from build123d import *

# Parameters (mm, degrees)
SKETCH_1_R      = 1.5
EXTRUDE_1_DEPTH = 1


with BuildPart() as part:
    # 草图1 → 凸台-拉伸1 (new body)
    with BuildSketch(Plane.XY):
        with BuildLine():
            ThreePointArc((9.027564348, -14.530044737), (9.452188044, -14.317284831), (9.814671703, -14.010401047))
            add(Edge.make_bspline(
                [(9.814671703, -14.010401047), (12.18822328, -11.458756692), (15.692863494, -5.893557839), (16.722450019, 0.624994049), (16.609112546, 4.098471157)],
                knots=[0.022064742, 0.022064742, 0.022064742, 0.022064742, 0.499959338, 0.977990906, 0.977990906, 0.977990906, 0.977990906], degree=3))
            ThreePointArc((16.609112546, 4.098471157), (16.53806505, 4.565454975), (16.359479137, 5.002752018))
            add(Edge.make_bspline(
                [(16.359479137, 5.002752018), (14.674806415, 8.042450428), (10.446892996, 13.109630634), (4.583537519, 16.088725104), (1.237093036, 17.061322309)],
                knots=[0.022009094, 0.022009094, 0.022009094, 0.022009094, 0.500040662, 0.977935258, 0.977935258, 0.977935258, 0.977935258], degree=3))
            ThreePointArc((1.237093036, 17.061322309), (0.768508115, 17.138783476), (0.294870912, 17.103571828))
            add(Edge.make_bspline(
                [(0.294870912, 17.103571828), (-3.125200659, 16.434385016), (-9.231172481, 13.992221488), (-13.895447236, 9.324238792), (-15.845236863, 6.448095314)],
                knots=[0.022064742, 0.022064742, 0.022064742, 0.022064742, 0.499960608, 0.977922402, 0.977922402, 0.977922402, 0.977922402], degree=3))
            ThreePointArc((-15.845236863, 6.448095314), (-16.062723303, 6.027327569), (-16.175163145, 5.567215485))
            add(Edge.make_bspline(
                [(-16.175163145, 5.567215485), (-16.595831692, 2.107197873), (-16.160161694, -4.45559692), (-13.161387867, -10.33481003), (-11.028034261, -13.078319909)],
                knots=[0.021996491, 0.021996491, 0.021996491, 0.021996491, 0.499960843, 0.977990945, 0.977990945, 0.977990945, 0.977990945], degree=3))
            ThreePointArc((-11.028034261, -13.078319909), (-10.696067568, -13.414360903), (-10.294548569, -13.663173939))
            add(Edge.make_bspline(
                [(-10.294548569, -13.663173939), (-7.144931204, -15.132114571), (-0.746064836, -16.746443383), (5.74855557, -15.710187793), (9.027564348, -14.530044737)],
                knots=[0.022009307, 0.022009307, 0.022009307, 0.022009307, 0.500040658, 0.977935258, 0.977935258, 0.977935258, 0.977935258], degree=3))
        make_face()
        with Locations((8.264326198, -12.518023506)):
            Circle(SKETCH_1_R, mode=Mode.SUBTRACT)
        with Locations((-9.351530584, -11.728123283)):
            Circle(SKETCH_1_R, mode=Mode.SUBTRACT)
        with Locations((-14.043889946, 5.269644693)):
            Circle(SKETCH_1_R, mode=Mode.SUBTRACT)
        with Locations((0.671929263, 14.984942812)):
            Circle(SKETCH_1_R, mode=Mode.SUBTRACT)
        with Locations((14.459165069, 3.991559284)):
            Circle(SKETCH_1_R, mode=Mode.SUBTRACT)
        with BuildLine():
            ThreePointArc((-12.084118167, 4.284259186), (-11.989009709, 4.498598439), (-11.919642267, 4.722596412))
            add(Edge.make_bspline(
                [(0.333250802, 12.818762133), (-2.935666702, 13.36550918), (-8.291080057, 12.535805727), (-11.122073794, 7.958530689), (-11.919642267, 4.722596412)],
                knots=[0.011876539, 0.011876539, 0.011876539, 0.011876539, 0.500003959, 0.988536873, 0.988536873, 0.988536873, 0.988536873], degree=3))
            ThreePointArc((0.333250802, 12.818762133), (0.573655745, 12.793365714), (0.815368633, 12.797159765))
            add(Edge.make_bspline(
                [(12.293898461, 3.640629682), (11.788818781, 6.932897703), (9.378560044, 11.743845098), (4.119958064, 13.049350775), (0.815368633, 12.797159765)],
                knots=[0.011651073, 0.011651073, 0.011651073, 0.011651073, 0.499978932, 0.988122793, 0.988122793, 0.988122793, 0.988122793], degree=3))
            ThreePointArc((12.293898461, 3.640629682), (12.343962742, 3.407799774), (12.421347321, 3.182571388))
            add(Edge.make_bspline(
                [(7.261467235, -10.567176253), (10.236427241, -9.069498048), (14.068062226, -5.28940284), (13.683697639, 0.116101841), (12.421347321, 3.182571388)],
                knots=[0.011651023, 0.011651023, 0.011651023, 0.011651023, 0.499963297, 0.988308236, 0.988308236, 0.988308236, 0.988308236], degree=3))
            ThreePointArc((7.261467235, -10.567176253), (7.05550434, -10.686738072), (6.865213221, -10.829933857))
            add(Edge.make_bspline(
                [(-7.806108488, -10.171458919), (-5.462403522, -12.538035871), (-0.683269899, -15.014043888), (4.338910959, -12.978090664), (6.865213221, -10.829933857)],
                knots=[0.011648007, 0.011648007, 0.011648007, 0.011648007, 0.499963567, 0.988308296, 0.988308296, 0.988308296, 0.988308296], degree=3))
            ThreePointArc((-7.806108488, -10.171458919), (-7.983418072, -10.012559189), (-8.178354084, -9.875855991))
            add(Edge.make_bspline(
                [(-12.084118167, 4.284259186), (-13.612076453, 1.322501907), (-14.491074702, -3.988767844), (-11.002068971, -8.136759896), (-8.178354084, -9.875855991)],
                knots=[0.011463127, 0.011463127, 0.011463127, 0.011463127, 0.499980132, 0.988311969, 0.988311969, 0.988311969, 0.988311969], degree=3))
        make_face(mode=Mode.SUBTRACT)
    extrude(amount=EXTRUDE_1_DEPTH)


solid = part.part
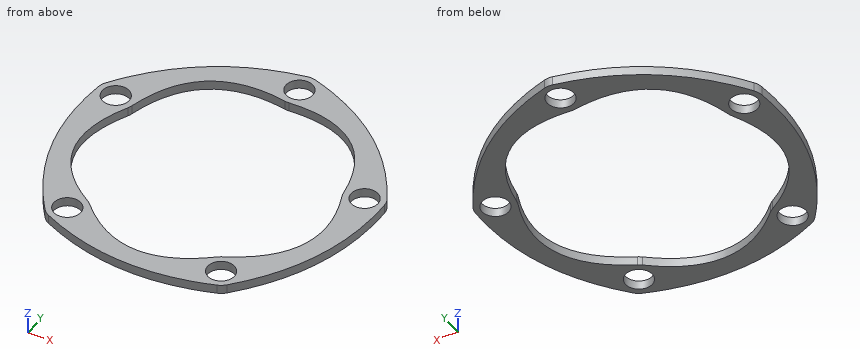
Design review of the part built by this model. Coordinates are the model's own, in mm. Give positions to 0.01 mm unless a question says otherwise; leave off trailing zeros. Use CSV: the item, a comma, the result in double quotes. Start each with the question number.
Q1. For line 1 (X direction, y = -10.5, z = 0.15); line 2 (X direction, y = 6.5, z = 0.8); line 3 (Y direction, x = -8.5, z = 0.9), list the stretches that pass through material, from the lowest coordinate up.
Q2. For P1, Ø2.5, axis at x = -14.04, y = 5.27, coming from the -Z side, flat-tipped, find the tip position at first contact; note if it passes through.
Q3. Take a section at A-A (z = 0.35). Count the separate pieces of the cut face and the enclosed holes in it, and give its area (3 significant figures).
Calculated:
1,line 1,"x = -12.81 to -10.21, -8.49 to -7.47, 7.39 to 12.59"
1,line 2,"x = -15.81 to -14.9, -13.19 to -11.39, 11.6 to 15.47"
1,line 3,"y = -14.43 to -12.96, -10.49 to -9.67, 10.96 to 13.68"
2,P1,"passes through"
3,separate pieces,"1"
3,enclosed holes,"6"
3,area,"248 mm²"
